from build123d import *

# Parameters (mm, degrees)
F0_R     = 32.5
F0_R_2   = 6
F0_R_3   = 5
F1_DEPTH = 5
F2_SIZE  = 0.5
F3_SIZE  = 0.5
F4_SIZE  = 0.5


with BuildPart() as f1:
    # F0 (on Front) → F1 (new body, symmetric)
    with BuildSketch(Plane.XZ):
        Circle(F0_R)
        with Locations((-11, -19.052559)):
            Circle(F0_R_2, mode=Mode.SUBTRACT)
        with Locations((11, -19.052559)):
            Circle(F0_R_2, mode=Mode.SUBTRACT)
        with Locations((-22, 0)):
            Circle(F0_R_2, mode=Mode.SUBTRACT)
        with Locations((-11, 19.052559)):
            Circle(F0_R_2, mode=Mode.SUBTRACT)
        Circle(F0_R_3, mode=Mode.SUBTRACT)
        with Locations((22, 0)):
            Circle(F0_R_2, mode=Mode.SUBTRACT)
        with Locations((11, 19.052559)):
            Circle(F0_R_2, mode=Mode.SUBTRACT)
    extrude(amount=F1_DEPTH, both=True)

    # F2
    f2_edges = [f1.edges().sort_by_distance(p)[0] for p in [
        (-32.5, -5, 0),
    ]]
    chamfer(f2_edges, length=F2_SIZE)

    # F3
    f3_edges = [f1.edges().sort_by_distance(p)[0] for p in [
        (5, 5, -19.052559),
        (5, -5, -19.052559),
        (16, 5, 0),
        (5, 5, 19.052559),
        (-32.5, 5, 0),
        (-17, 5, 19.052559),
        (-28, 5, 0),
        (-17, 5, -19.052559),
        (16, -5, 0),
        (5, -5, 19.052559),
        (-17, -5, 19.052559),
        (-17, -5, -19.052559),
    ]]
    chamfer(f3_edges, length=F3_SIZE)

    # F4
    f4_edges = [f1.edges().sort_by_distance(p)[0] for p in [
        (-28, -5, 0),
    ]]
    chamfer(f4_edges, length=F4_SIZE)


solid = f1.part
Source: CAD feature listing. Evaluate the final solid. Frame: model axes, mm. Round coordinates to 2 decimals unless told otherwise and drop trailing zeros. Loops run counter-clockwise (first coordinate to the right, second up) from the corner with the lowest first, then second, coordinate; pieces in that order, holes last.
Q1. Section D-D, the plane x = -11. State how many separate pieces and enclosed holes the cut face has, plus the area to 3 significant figures.
Q2. Ray query, line 1 (Z direction, x = -6, y = -4.25); line 2 (X direction, y = -4, z = -23.5); line 3 (X direction, y = 3.5, z = -14). Return the intervals inside material, ascending.
Q3. First-contact query: P1, Ø3, axis at x = 9, y = 2.5, coming from the +Z side; P2, Ø4, axis at y = 1, z = 21, coming from the +X side; P3, Ø4, axis at x = -10, y = 1, coming from the -Z side. Flat tips, straight axial feed; report the tip coordinate or a pass-through.
Q4. Mould query, pull axis Z, two halves, no side actions, for faces 1 (the face through (-26.76, 0.06, -3.65)), 2 (the face through (-7.774, 0.063, -13.993)), 3 (the face through (0, -5, -7)). Classes: pulls with the +Z half, pulls with the -Z half, needs draft (parallel to the pull), parting line crosses it, or undercut.
Q5. Section B-B, the plane z = 0. Return loops of the section in (x, y).
Q6. Section A-A, the plane x = 0. Return loops of the section in (y, z).
Q7. Section C-C, the plane y = 3.5. Return loops of the section in (x, z).
Solutions:
1. separate pieces: 3
1. enclosed holes: 0
1. area: 370 mm2
2. line 1: z = -31.94 to -22.37, -15.74 to 15.74, 22.37 to 31.94
2. line 2: x = -22.45 to -15.03, -6.97 to 6.97, 15.03 to 22.45
2. line 3: x = -29.33 to -14.24, -7.76 to 7.76, 14.24 to 29.33
3. P1: stops at z = 31.62
3. P2: stops at x = 26.37
3. P3: stops at z = -31.5
4. face 1: undercut
4. face 2: undercut
4. face 3: needs draft
5. outline: (-32.5, -4.5) - (-32, -5) - (-28.5, -5) - (-28, -4.5) - (-28, 4.5) - (-28.5, 5) - (-32, 5) - (-32.5, 4.5) - close; (-16, -4.5) - (-15.5, -5) - (-5, -5) - (-5, 5) - (-15.5, 5) - (-16, 4.5) - close; (5, -5) - (15.5, -5) - (16, -4.5) - (16, 4.5) - (15.5, 5) - (5, 5) - close; (28, -4.5) - (28.5, -5) - (32, -5) - (32.5, -4.5) - (32.5, 4.5) - (32, 5) - (28.5, 5) - (28, 4.5) - close
6. outline: (-5, -32) - (-4.5, -32.5) - (4.5, -32.5) - (5, -32) - (5, -5) - (-5, -5) - close; (-5, 5) - (5, 5) - (5, 32) - (4.5, 32.5) - (-4.5, 32.5) - (-5, 32) - close
7. outline: circle Ø65 at (0, 0); hole circle Ø12 at (-22, 0); hole circle Ø12 at (-11, -19.05); hole circle Ø12 at (-11, 19.05); hole circle Ø10 at (0, 0); hole circle Ø12 at (11, -19.05); hole circle Ø12 at (11, 19.05); hole circle Ø12 at (22, 0)
